Geometry: final body of the model. Coordinates: model frame, mm. Face numbers are marked on the shaded views. A direction names the side the tool comes from. Give positions to 0.01 mm unless a question says otherwise; leave off trailing zeros. Write each loop counter-clockwise with the first axis right and the second up, starting at its lowest first coordinate (ties: lowest second). Pieces come first, ordered by that corner, then holes. Notation, with made-up numbers: (16, -31) - (37, -31) arc R31 ccw to (37, -4) - close; hole circle Ø4 at (-16, -15). An arc over 180 degrees is marked (long way). Return JSON: item names as keys, results as strings.
Autodesk Inventor part; units mm, degrees
ref_plane "YZ Plane" through (0, 0, 0) normal (1, 0, 0) x (0, 1, 0)
ref_plane "XZ Plane" through (0, 0, 0) normal (0, 1, 0) x (-1, 0, 0)
ref_plane "XY Plane" through (0, 0, 0) normal (0, 0, 1) x (1, 0, 0)
sketch "Sketch1" plane through (0, 0, 0) normal (0, 0, 1) x (1, 0, 0)
  line L0 (12, 0) -> (64, 0)
  line L1 (64, 0) -> (64, 71.9)
  line L2 (64, 71.9) -> (0, 71.9)
  line L3 (0, 71.9) -> (0, 12)
  line L4 (3, 65.9) -> (9, 65.9)
  line L5 (9, 65.9) -> (9, 57.9)
  line L6 (9, 57.9) -> (3, 57.9)
  line L7 (3, 57.9) -> (3, 65.9)
  line L8 (3, 42.9) -> (9, 42.9)
  line L9 (9, 42.9) -> (9, 34.9)
  line L10 (9, 34.9) -> (3, 34.9)
  line L11 (3, 34.9) -> (3, 42.9)
  line L12 (0, 12) -> (12, 12)
  line L13 (12, 12) -> (12, 0)
  line L14 (3, 57.9) -> (9, 42.9) construction
  line L15 (3, 42.9) -> (9, 57.9) construction
  circle A0 centre (6, 50.4) radius 2.25
  point P0 (0, 0)
  dimension "d1" = 6
  dimension "d2" = 8
  dimension "d3" = 8
  dimension "d4" = 15
  dimension "d5" = 3
  dimension "d6" = 71.9
  dimension "d7" = 4.5
  dimension "d8" = 64
  dimension "d9" = 12
  dimension "d10" = 52
  dimension "d11" = 6
extrude "Extrusion1" add sketch "Sketch1" along normal blind 6
sketch "Sketch2" plane through (0, 0, 6) normal (0, 0, 1) x (1, 0, 0)
  line L0 (64, 0) -> (64, 71.9)
  line L1 (12, 0) -> (64, 0)
  line L2 (29.75, 16.3) -> (34.25, 16.3)
  line L3 (34.25, 0) -> (29.75, 0)
  line L4 (36.75, 12.3) -> (36.75, 5)
  line L5 (27.25, 5) -> (27.25, 12.3)
  line L6 (29.75, 0) -> (29.75, 5)
  line L7 (29.75, 12.3) -> (29.75, 16.3)
  line L8 (27.25, 12.3) -> (29.75, 12.3)
  line L9 (34.25, 12.3) -> (36.75, 12.3)
  line L10 (34.25, 16.3) -> (34.25, 12.3)
  line L11 (34.25, 5) -> (34.25, 0)
  line L12 (36.75, 5) -> (34.25, 5)
  line L13 (29.75, 5) -> (27.25, 5)
  point P0 (0, 0)
  point P1 (32, 16.3)
  dimension "d14" = 2.5
  dimension "d15" = 2.5
  dimension "d16" = 4.5
  dimension "d17" = 5
  dimension "d18" = 7.3
  dimension "d19" = 4
  dimension "d20" = 32
extrude "Extrusion2" cut sketch "Sketch2" against normal blind 6
sketch "Sketch3" plane through (0, 0, 6) normal (0, 0, 1) x (1, 0, 0)
  line L0 (34.25, 0) -> (64, 0)
  line L1 (12, 0) -> (29.75, 0)
  line L2 (29.75, 16.3) -> (34.25, 16.3)
  line L3 (16.5, 0) -> (24.5, 0)
  line L4 (24.5, 0) -> (24.5, -4)
  line L5 (22.5, -6) -> (18.5, -6)
  line L6 (16.5, -4) -> (16.5, 0)
  line L7 (39.5, 0) -> (47.5, 0)
  line L8 (47.5, 0) -> (47.5, -4)
  line L9 (45.5, -6) -> (41.5, -6)
  line L10 (39.5, -4) -> (39.5, 0)
  arc A0 (16.5, -4) -> (18.5, -6) centre (18.5, -4) ccw
  arc A1 (22.5, -6) -> (24.5, -4) centre (22.5, -4) ccw
  arc A2 (39.5, -4) -> (41.5, -6) centre (41.5, -4) ccw
  arc A3 (45.5, -6) -> (47.5, -4) centre (45.5, -4) ccw
  point P0 (0, 0)
  point P1 (32, 16.3)
  dimension "d23" = 2
  dimension "d24" = 8
  dimension "d25" = 8
  dimension "d26" = 6
  dimension "d27" = 15
  dimension "d28" = 7.5
extrude "Extrusion3" add sketch "Sketch3" against normal blind 6
chamfer "Chamfer1" distance 2 angle 45 2 edges at (0, 71.9, 3) (64, 71.9, 3)
sketch "Sketch4" plane through (0, 0, 0) normal (0, 0, -1) x (-1, 0, 0)
  line L0 (-64, 69.9) -> (-64, 0)
  line L1 (-2, 71.9) -> (-62, 71.9)
  line L2 (-39, 58.9) -> (-53, 58.9)
  line L3 (-53, 58.9) -> (-53, 44.9)
  line L4 (-53, 44.9) -> (-39, 44.9)
  line L5 (-39, 44.9) -> (-39, 58.9)
  line L6 (-34, 65.9) -> (-58, 65.9) construction
  line L7 (-58, 65.9) -> (-58, 37.9) construction
  line L8 (-58, 37.9) -> (-34, 37.9) construction
  line L9 (-34, 37.9) -> (-34, 65.9) construction
  circle A0 centre (-58, 60.9) radius 1.6
  circle A1 centre (-58, 42.9) radius 1.6
  circle A2 centre (-53, 37.9) radius 1.6
  circle A3 centre (-39, 37.9) radius 1.6
  circle A4 centre (-34, 42.9) radius 1.6
  circle A5 centre (-34, 60.9) radius 1.6
  circle A6 centre (-39, 65.9) radius 1.6
  circle A7 centre (-53, 65.9) radius 1.6
  point P0 (0, 0)
  point P1 (-58, 51.9)
  point P2 (-53, 51.9)
  point P3 (-46, 37.9)
  point P4 (-46, 44.9)
  dimension "d34" = 3.2
  dimension "d35" = 5
  dimension "d36" = 5
  dimension "d37" = 5
  dimension "d38" = 5
  dimension "d39" = 5
  dimension "d40" = 5
  dimension "d41" = 5
  dimension "d42" = 5
  dimension "d43" = 14
  dimension "d44" = 14
  dimension "d45" = 5
  dimension "d46" = 7
  dimension "d47" = 6
  dimension "d48" = 6
extrude "Extrusion4" cut sketch "Sketch4" against normal through all
chamfer "Chamfer2" distance 2 angle 45 2 edges at (0, 12, 3) (12, 12, 3)
equation "\"d36\" = d35"
equation "\"d37\" = d35"
equation "\"d38\" = d35"
equation "\"d39\" = d35"
equation "\"d40\" = d35"
equation "\"d41\" = d35"
equation "\"d42\" = d35"
properties part number "x_motor_cable_mount"
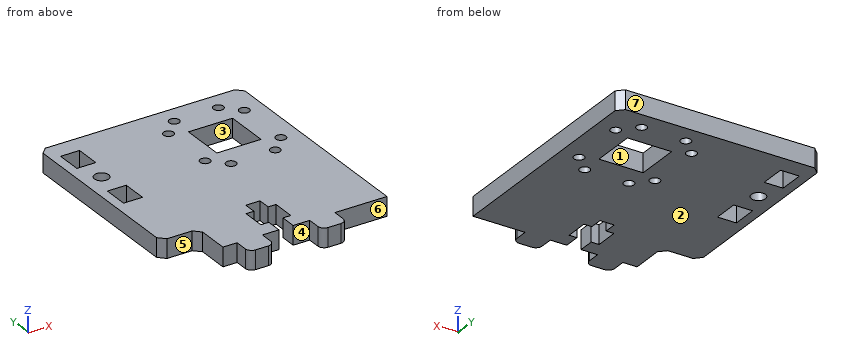
Q1. Set-up query: the marked faces 3, 4, 5, 6 and 7. Return all of +Z, -Z, +X, -X, +Y, -Y with unobstructed straight access to the full face (end or side cutting, diameter ignored); none if empty.
Answer key:
{"face 3": "+Z, -Z", "face 4": "+Z, -Z, -Y", "face 5": "+Z, -Z, -X, -Y", "face 6": "+Z, -Z, +X, -Y", "face 7": "+Z, -Z, +X, -X, +Y"}
Q2. Material intervals for probe 1 along Y at (x, z) = (34, 4.5); probe 2 along Y at (x, z) = (6, 2.2); probe 3 along X at (y, z) = (58, 0.4), sorted ascending. Write a range as [from, to].
Answer key:
{"probe 1": "y = [16.3, 41.3], [44.5, 59.3], [62.5, 71.9]", "probe 2": "y = [12, 34.9], [42.9, 48.15], [52.65, 57.9], [65.9, 71.9]", "probe 3": "x = [0, 3], [9, 39], [53, 64]"}
Q3. Section query C-C, the plane y = 2.5. Return the cut outline in (x, z), plus the area to 3 significant figures.
Answer key:
{"outline": "(12, 0) - (29.75, 0) - (29.75, 6) - (12, 6) - close; (34.25, 0) - (64, 0) - (64, 6) - (34.25, 6) - close", "area": "285 mm^2"}
Q4. Section query A-A, the plane x = 58. Return the cut outline in (y, z).
Answer key:
{"outline": "(0, 0) - (41.3, 0) - (41.3, 6) - (0, 6) - close; (44.5, 0) - (59.3, 0) - (59.3, 6) - (44.5, 6) - close; (62.5, 0) - (71.9, 0) - (71.9, 6) - (62.5, 6) - close"}
Q5. Pin query (flat end, axial travel): P1, Ø1.8, axis at x = 7, z = 3, coming from the -Y side; P2, Ø1.9, axis at x = 34, y = 60.9, coming from the -Z side; P3, Ø2, axis at y = -1.5, z = 4, coming from the -X side; P4, Ø2, axis at y = -1.5, z = 2, coming from the +X side. Return the tip coordinate at first contact, or that it passes through.
Answer key:
{"P1": "stops at y = 12", "P2": "passes through", "P3": "stops at x = 16.5", "P4": "stops at x = 47.5"}
Q6. Section query B-B, the plane y = 37.9. Return the cut outline in (x, z), plus the area to 3 significant figures.
Answer key:
{"outline": "(0, 0) - (3, 0) - (3, 6) - (0, 6) - close; (9, 0) - (37.4, 0) - (37.4, 6) - (9, 6) - close; (40.6, 0) - (51.4, 0) - (51.4, 6) - (40.6, 6) - close; (54.6, 0) - (64, 0) - (64, 6) - (54.6, 6) - close", "area": "310 mm^2"}
Q7. Section query D-D, the plane z = 1.75. Count the separate pieces of the cut face and the enclosed holes in it, plus the area to 3 significant figures.
Answer key:
{"separate pieces": "1", "enclosed holes": "12", "area": "4,060 mm^2"}
Q8. Mould query, pull axis X, two halves, no side actions, for the marked faces 1 and 2. Classes: pulls with the +X half, pulls with the -X half, needs draft (parallel to the pull), parting line crosses it, or undercut.
Answer key:
{"face 1": "undercut", "face 2": "needs draft"}
